Input: part model. Units: mm. Frame: model coordinates. Face numbers are marked on the shaded views. A direction names the side the tool comes from. Give positions to 0.01 mm unless a question says otherwise; leave off trailing zeros. Write each loop counter-clockwise with the first axis right and the second up, starting at its lowest first coordinate (ties: lowest second). Pieces come first, ordered by that corner, then holes.
Autodesk Fusion 360 part; units mm, degrees
sketch "Sketch1" plane through (0, 0, 0) normal (0, 0, 1) x (1, 0, 0)
  circle A0 centre (0, 0) radius 30.4
  circle A1 centre (0, 0) radius 33.4
  circle A2 centre (0, 0) radius 36.4
  circle A3 centre (0, 0) radius 7.5
  circle A4 centre (0, 0) radius 14
  line L0 (0, 0) -> (4.7883, -13.1557)
  line L1 (0, 0) -> (-4.7883, -13.1557)
  line L2 (0, -60) -> (0, 60)
  line L3 (4.7883, -13.1557) -> (8.5505, -23.4923)
  line L4 (-4.7883, -13.1557) -> (-8.5505, -23.4923)
  arc A5 (8.5505, -23.4923) -> (-8.5505, -23.4923) centre (0, 0) ccw
  arc A6 (-8.5505, -23.4923) -> (0, -25) centre (0, 0) ccw
  arc A7 (0, -25) -> (8.5505, -23.4923) centre (0, 0) ccw
  line L5 (13.7873, -2.4311) -> (24.6202, -4.3412)
  line L6 (8.999, -10.7246) -> (16.0697, -19.1511)
  line L7 (8.999, 10.7246) -> (16.0697, 19.1511)
  line L8 (13.7873, 2.4311) -> (24.6202, 4.3412)
  line L9 (-4.7883, 13.1557) -> (-8.5505, 23.4923)
  line L10 (4.7883, 13.1557) -> (8.5505, 23.4923)
  line L11 (-13.7873, 2.4311) -> (-24.6202, 4.3412)
  line L12 (-8.999, 10.7246) -> (-16.0697, 19.1511)
  line L13 (-8.999, -10.7246) -> (-16.0697, -19.1511)
  line L14 (-13.7873, -2.4311) -> (-24.6202, -4.3412)
  circle A8 centre (0, 0) radius 3.5
  circle A9 centre (0, 0) radius 5.5
  point P0 (0, 7.5)
  dimension "d1" = 60.8
  dimension "d2" = 3
  dimension "d3" = 3
  dimension "d4" = 15
  dimension "d11" = 28
  dimension "d12" = 50
  dimension "d13" = 40
  dimension "d15" = 20
  dimension "d17" = 360
  dimension "d22" = -4
  dimension "d34" = -2
extrude "Extrude1" add sketch "Sketch1" against normal blind 10 contours A0 A1 L2 | A0 A1 L2
extrude "Extrude2" add sketch "Sketch1" along normal blind 3 contours A0 L2 A5 A7 | A0 A1 L2 | A0 L2 A5 A6 | A0 A1 L2 | A4 L2 A5 L10 | A4 L2 A5 L9 | A1 A2 L2 | A1 A2 L2 | A4 L2 L4 A6 | A4 L2 L3 A7 | A3 A4 L1 L2 | A3 A4 L0 L2 | A4 A5 L7 L10 | A4 A5 L9 L12 | A3 A4 L0 L2 | A3 A4 L1 L2 | A4 L4 A5 L13 | A4 L3 A5 L6 | A4 A5 L7 L8 | A4 A5 L11 L12 | A4 A5 L13 L14 | A4 A5 L5 L6 | A4 A5 L5 L8 | A4 A5 L11 L14
extrude "Extrude3" add sketch "Sketch1" along normal blind 25 contours A3 L1 L2 A9 | A3 L0 L2 A9 | A3 L0 L2 A9 | A3 L1 L2 A9 | L0 L2 A8 A9 | L1 L2 A8 A9 | L1 L2 A8 A9 | L0 L2 A8 A9 | L0 L2 A8 | L1 L2 A8 | L1 L2 A8 | L0 L2 A8
extrude "Extrude4" cut sketch "Sketch1" along normal blind 3 contours A4 L2 A5 L10 | A4 L2 A5 L9 | A4 L2 L4 A6 | A4 L2 L3 A7 | A4 A5 L7 L8 | A4 A5 L11 L12 | A4 A5 L13 L14 | A4 A5 L5 L6
fillet "Fillet1" radius 4 24 edges at (-16.0697, 19.1511, 1.5) (-24.6202, 4.3412, 1.5) (-13.7873, 2.4311, 1.5) (-8.999, 10.7246, 1.5) (-13.7873, -2.4311, 1.5) (-24.6202, -4.3412, 1.5) (-16.0697, -19.1511, 1.5) (-8.999, -10.7246, 1.5) (-4.7883, -13.1557, 1.5) (-8.5505, -23.4923, 1.5) (8.5505, -23.4923, 1.5) (4.7883, -13.1557, 1.5) (8.999, -10.7246, 1.5) (16.0697, -19.1511, 1.5) (24.6202, -4.3412, 1.5) (13.7873, -2.4311, 1.5) (24.6202, 4.3412, 1.5) (16.0697, 19.1511, 1.5) (13.7873, 2.4311, 1.5) (8.999, 10.7246, 1.5) (4.7883, 13.1557, 1.5) (8.5505, 23.4923, 1.5) (-4.7883, 13.1557, 1.5) (-8.5505, 23.4923, 1.5)
extrude "Extrude5" cut sketch "Sketch1" against normal up to surface (22 mm away) from surface at 25 contours L0 L2 A8 | L1 L2 A8 | L1 L2 A8 | L0 L2 A8
extrude "Extrude7" cut sketch "Sketch1" along normal blind 7 from surface at 9 contours A3 L1 L2 A9 | A3 L0 L2 A9 | A3 L0 L2 A9 | A3 L1 L2 A9
fillet "Fillet4" radius 4 1 edges at (-6.9925, -2.7121, 25)
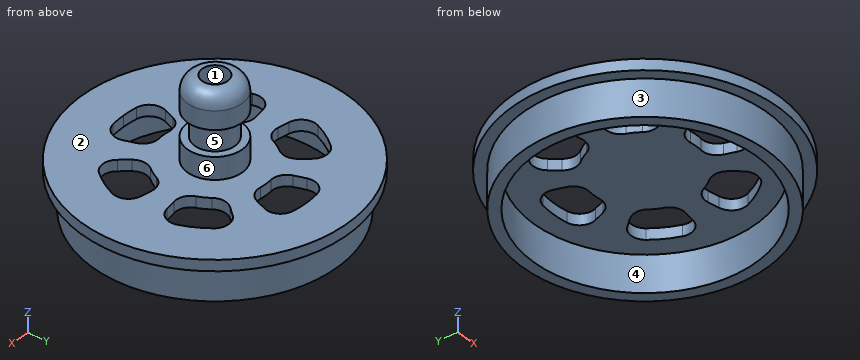
Item 1: Section D-D (y = 6.5). Give the number of separate pieces and of enclosed holes in the cut face, and give its area (3 significant figures).
Item 2: Pin query (flat end, axial travel): pin 1 (1 mm diameter, centred on y = -12, z = -4.5, fed in from +X); pin 2 (1 mm diameter, centred on y = 24, z = 0, fed in from -X); pin 3 (8 mm diameter, centred on x = -0.5, z = 11, fed in from +Y). Return the tip coordinate at first contact, or that it passes through.
Item 3: Ray query, line 1 (X direction, y = 0, z = -5.5); line 2 (Y direction, x = 0, z = 13.5); line 3 (Y direction, x = 0, z = 19). Return the intervals inside material, ascending.
Item 4: Section B-B (y = 21). Return loops of the section in (x, z), and give its area (3 significant figures).
Item 5: Set-up query: the marked faces 4, 5 and 6. Return all of +Z, -Z, +X, -X, +Y, -Y with unobstructed straight access to the full face (end or side cutting, diameter ignored); none if empty.
Item 6: Section A-A (z = 13). Return loops of the section in (x, y), and give its area (3 significant figures).
Item 7: Mould query, pull axis X, two halves, no side actions, for the marked faces 1, 2 and 3. Classes: +X half, -X half, draft (parallel to the pull), parting line (faces both ways), or undercut.
Item 8: Section C-C (x = 24.5). Return loops of the section in (y, z).
Solved:
1. separate pieces: 4
1. enclosed holes: 0
1. area: 308 mm2
2. pin 1: stops at x = 31.36
2. pin 2: stops at x = -27.8
2. pin 3: stops at y = 7.5
3. line 1: x = -33.4 to -30.4, 30.4 to 33.4
3. line 2: y = -5.5 to -3.5, 3.5 to 5.5
3. line 3: y = -7.5 to -3.5, 3.5 to 7.5
4. outline: (-29.73, 0) - (-25.97, 0) - (-25.97, -10) - (-21.98, -10) - (-21.98, 0) - (-7.28, 0) - (-7.28, 3) - (-29.73, 3) - close; (7.28, 0) - (21.98, 0) - (21.98, -10) - (25.97, -10) - (25.97, 0) - (29.73, 0) - (29.73, 3) - (7.28, 3) - close
4. area: 215 mm2
5. face 4: -Z
5. face 5: none
5. face 6: +Z
6. outline: circle Ø11 at (0, 0); hole circle Ø7 at (0, 0)
6. area: 56.5 mm2
7. face 1: undercut
7. face 2: draft
7. face 3: parting line
8. outline: (-26.92, 0) - (-22.7, 0) - (-22.7, -10) - (-18, -10) - (-18, 0) - (18, 0) - (18, -10) - (22.7, -10) - (22.7, 0) - (26.92, 0) - (26.92, 3) - (-26.92, 3) - close
